from build123d import *

# Parameters (mm, degrees)
F0_R     = 5
F1_DEPTH = 10


with BuildPart() as f1:
    # F0 (on Top) → F1 (new body)
    with BuildSketch(Plane.XY):
        with BuildLine():
            ThreePointArc((55, 0), (52.071068, 7.071068), (45, 10))
            Line((45, 10), (-45, 10))
            ThreePointArc((-45, 10), (-52.071068, 7.071068), (-55, 0))
            ThreePointArc((-55, 0), (-52.071068, -7.071068), (-45, -10))
            Line((-45, -10), (45, -10))
            ThreePointArc((45, -10), (52.071068, -7.071068), (55, 0))
        make_face()
        with Locations((-45, 0)):
            Circle(F0_R, mode=Mode.SUBTRACT)
        with Locations((45, 0)):
            Circle(F0_R, mode=Mode.SUBTRACT)
    extrude(amount=F1_DEPTH)


solid = f1.part
Geometry check sheet. Reference: the model listing, model coordinates, mm. Round coordinates to 2 decimals unless told otherwise and drop trailing zeros. Order: outer loops, then holes, each group sorted by start corner. A loop starts at its lowest first (then second) coordinate and runs counter-clockwise, first axis right, second up. Notation, with made-up numbers: (-0.5, 43.25) -> (49.5, 43.25) arc R13 ccw to (49.5, 54.25) -> close; hole circle Ø10 at (83.25, -17). An arc over 180 degrees is marked (long way). Use one line per item in the form item = value.
1. Cross-section at A-A, the plane z = 2.5. Enter the section's corners in (x, y), plus the area to 3 significant figures.
Working result:
outline = (-55, 0) arc R10 ccw to (-45, -10) -> (45, -10) arc R10 ccw to (55, 0) arc R10 ccw to (45, 10) -> (-45, 10) arc R10 ccw to start; hole circle Ø10 at (-45, 0); hole circle Ø10 at (45, 0)
area = 1,960 mm^2
2. Scan lines: line 1 along X through (y, z) = (-0.25, 7.5); line 2 along Y through (x, z) = (45, 7.25); line 3 along X through (y, z) = (-4, 3.25). Record each from-to range of solid material in increasing order. Write a range as from..to.
Working result:
line_1 = -55..-49.99, -40.01..40.01, 49.99..55
line_2 = -10..-5, 5..10
line_3 = -54.17..-48, -42..42, 48..54.17
3. Cross-section at C-C, the plane y = 8.25. Enter the section's corners in (x, z), plus the area to 3 significant figures.
Working result:
outline = (-50.65, 0) -> (50.65, 0) -> (50.65, 10) -> (-50.65, 10) -> close
area = 1,010 mm^2
4. Go/stop test with flat-tipped pins: pin 1 (1 mm diameter, centred on y = 4, z = 5, fed in from -X); pin 2 (3 mm diameter, centred on y = 6.5, z = 7, fed in from -X). Record where each tip stops, or that it passes through.
Working result:
pin_1 = -54.37
pin_2 = -53.66
5. Cross-section at B-B, the plane x = -46.5. Enter the section's corners in (y, z).
Working result:
outline = (-9.89, 0) -> (-4.77, 0) -> (-4.77, 10) -> (-9.89, 10) -> close; (4.77, 0) -> (9.89, 0) -> (9.89, 10) -> (4.77, 10) -> close
6. Mould release check, pull along X, two halves, no side actions. Record for faces 1 (the face through (-1, 0, 0)), 2 (the face through (-50, 0, 5)), 3 (the face through (40, 0, 5)): pulls with the +X half, pulls with the -X half, needs draft (parallel to the pull), parting line crosses it, or undercut.
Working result:
face_1 = needs draft
face_2 = undercut
face_3 = undercut
